from build123d import *
from OCP.BRepFilletAPI import BRepFilletAPI_MakeChamfer

# Parameters (mm, degrees)
SKETCH1_W           = 65
SKETCH1_H           = 64
SKETCH1_W_2         = 44.2
SKETCH1_H_2         = 40
BOSS_EXTRUDE1_DEPTH = 15
SKETCH3_W           = 7
SKETCH3_H           = 11.1
SKETCH4_R           = 9.5
CUT_EXTRUDE2_DEPTH  = 74.986485252
SKETCH5_R           = 4
CUT_EXTRUDE3_DEPTH  = 74.32973476
SKETCH8_R           = 2.15
CUT_EXTRUDE6_DEPTH  = 49.013019068
FILLET1_R           = 20
CHAMFER1_SIZE       = 3
CHAMFER1_SIZE2      = 1.732050808
SKETCH9_W           = 12
SKETCH9_H           = 3


with BuildPart() as part:
    # Sketch1 → Boss-Extrude1 (new body)
    with BuildSketch(Plane(origin=(0, 0, 0), x_dir=(1, 0, 0), z_dir=(0, 1, 0))):
        Rectangle(SKETCH1_W, SKETCH1_H)
        Rectangle(SKETCH1_W_2, SKETCH1_H_2, mode=Mode.SUBTRACT)
    extrude(amount=BOSS_EXTRUDE1_DEPTH)

    # Sketch3 → Cut-Revolve1 (revolve, cut)
    with BuildSketch(Plane(origin=(0, 15, 0), x_dir=(1, 0, 0), z_dir=(0, 1, 0))):
        with Locations((25.6, -5.55)):
            Rectangle(SKETCH3_W, SKETCH3_H)
        with Locations((-25.6, -5.55)):
            Rectangle(SKETCH3_W, SKETCH3_H)
    revolve(axis=Axis((22.1, 15, 0), (1, 0, 0)), mode=Mode.SUBTRACT)

    # Sketch4 → Cut-Extrude2 (cut, through all)
    with BuildSketch(Plane(origin=(32.5, 0, 0), x_dir=(0, 0, -1), z_dir=(1, 0, 0))):
        with Locations((0, 15)):
            Circle(SKETCH4_R)
    extrude(amount=-CUT_EXTRUDE2_DEPTH, mode=Mode.SUBTRACT)

    # Sketch5 → Cut-Extrude3 (cut, through all)
    with BuildSketch(Plane.XY.offset(32)):
        with Locations((0, 15)):
            Circle(SKETCH5_R)
    extrude(amount=-CUT_EXTRUDE3_DEPTH, mode=Mode.SUBTRACT)

    # Sketch8 → Cut-Extrude6 (cut, through all)
    with BuildSketch(Plane(origin=(0, 15, 0), x_dir=(1, 0, 0), z_dir=(0, 1, 0))):
        with Locations((18, 16.5)):
            Circle(SKETCH8_R)
        with Locations((18, -16.5)):
            Circle(SKETCH8_R)
        with Locations((-18, -16.5)):
            Circle(SKETCH8_R)
        with Locations((-18, 16.5)):
            Circle(SKETCH8_R)
        with Locations(Location((9, -27, 0), (0, 0, 270))):
            Circle(SKETCH8_R)
        with Locations(Location((-9, -27, 0), (0, 0, 270))):
            Circle(SKETCH8_R)
        with Locations(Location((-9, 27, 0), (0, 0, 270))):
            Circle(SKETCH8_R)
        with Locations(Location((9, 27, 0), (0, 0, 270))):
            Circle(SKETCH8_R)
    extrude(amount=-CUT_EXTRUDE6_DEPTH, mode=Mode.SUBTRACT)

    # Fillet1
    fillet1_edges = [part.edges().sort_by_distance(p)[0] for p in [
        (-32.5, 7.5, -32),
        (32.5, 7.5, -32),
        (32.5, 7.5, 32),
        (-32.5, 7.5, 32),
    ]]
    fillet(fillet1_edges, radius=FILLET1_R)

    # Chamfer1: one chamfer whose edges measure the first distance from different faces: ONE call of the kernel's chamfer builder (chamfer() names one face for all edges)
    chamfer1_edges_1 = [part.edges().sort_by_distance(p)[0] for p in [
        (22.1, 3.9, 0),
    ]]
    chamfer1_side_1 = [part.faces().sort_by_distance(p)[0] for p in [
        (22.1, 0.427200187, 0),
    ]]
    chamfer1_edges_2 = [part.edges().sort_by_distance(p)[0] for p in [
        (-22.1, 3.9, 0),
    ]]
    chamfer1_side_2 = [part.faces().sort_by_distance(p)[0] for p in [
        (-22.1, 0.427200187, 0),
    ]]
    chamfer1 = BRepFilletAPI_MakeChamfer(part.part.solid().wrapped)
    for e in chamfer1_edges_1:
        chamfer1.Add(CHAMFER1_SIZE, CHAMFER1_SIZE2, e.wrapped, chamfer1_side_1[0].wrapped)  # the first distance lies on this face
    for e in chamfer1_edges_2:
        chamfer1.Add(CHAMFER1_SIZE, CHAMFER1_SIZE2, e.wrapped, chamfer1_side_2[0].wrapped)  # the first distance lies on this face
    add(Compound.cast(chamfer1.Shape()), mode=Mode.REPLACE)

    # Sketch9 → Cut-Revolve2 (revolve, cut)
    with BuildSketch(Plane(origin=(0, 15, 0), x_dir=(1, 0, 0), z_dir=(0, 1, 0))):
        with Locations((-6, -21.5)):
            Rectangle(SKETCH9_W, SKETCH9_H)
        with Locations((-6, 21.5)):
            Rectangle(SKETCH9_W, SKETCH9_H)
    revolve(axis=Axis((0, 15, -29.871415895), (0, 0, 1)), mode=Mode.SUBTRACT)


solid = part.part
Geometry: final body of the model. Coordinates: model frame, mm. A direction names the side the tool comes from. Give positions to 0.01 mm unless a question says otherwise; leave off trailing zeros. Write each loop counter-clockwise with the first axis right and the second up, starting at its lowest first coordinate (ties: lowest second). Pieces come first, ordered by that corner, then holes. Notation, with made-up numbers: M 55,48 L 110,48 A27 ccw 110,79 Z; hole C 11,49 d7. An arc over 180 degrees is marked long. Answer in a Markdown table with one row per item. Add a question column.
(1) Section C-C on x = 9. Return loops of the section in (y, z).
(2) Section A-A on z = 0. Return loops of the section in (x, y), and give its area (3 significant figures).
(3) Section D-D on z = 27. Return loops of the section in (x, y), and give its area (3 significant figures).
(4) First-contact query: pin 1 (5.5 mm diameter, centred on x = 9, z = 27, fed in from +Y); pin 2 (3 mm diameter, centred on x = -16.5, y = 11, fed in from -Z); pin 3 (2 mm diameter, centred on x = -19.5, y = 5.5, fed in from -Z); pin 4 (2 mm diameter, centred on x = -24.5, y = 7, fed in from -Z). Flat tips, straight axial feed; report the tip coordinate or a pass-through.
(5) Reachability of faces 1 (the flat face through (0, 2, -20)), 2 (the flat face through (0, 7, -32)), 3 (the flat face through (29.1, 5, 0)) from +Z, -Z, +X, -X, +Y, -Y: full face, straight path, thin tool, end or side. Return the list, or none.
(6) Section B-B on x = 0. Return loops of the section in (y, z).
(7) Ray query, line 1 (Z direction, x = 1, y = 7.75); line 2 (X direction, y = 7.25, z = 27); line 3 (X direction, y = 8, z = 27.5). Return the intervals inside material, ascending.
(8) Mould query, pull axis Z, two halves, no side actions, for faces 4 (the flat face through (-18, 15, 23)), 5 (the cylindrical face through (26.486, 7.605, 26.297)), 6 (the cylindrical face through (11.13, 7.6, -27.28)). Classes: +Z half, -Z half, draft (parallel to the pull), parting line (faces both ways), or undercut.
Result set:
| question | item | result |
|---|---|---|
| 1 | outline | M 0,-32 L 15,-32 L 15,-29.15 L 0,-29.15 Z; M 0,-24.85 L 15,-24.85 L 15,-23 L 7.06,-23 L 7.06,-20 L 0,-20 Z; M 0,20 L 7.06,20 L 7.06,23 L 15,23 L 15,24.85 L 0,24.85 Z; M 0,29.15 L 15,29.15 L 15,32 L 0,32 Z |
| 2 | outline | M -32.5,0 L -22.1,0 L -22.1,0.9 L -23.83,3.9 L -29.1,3.9 L -29.1,5.5 L -32.5,5.5 Z; M 22.1,0 L 32.5,0 L 32.5,5.5 L 29.1,5.5 L 29.1,3.9 L 23.83,3.9 L 22.1,0.9 Z |
| 2 | area | 86.8 mm^2 |
| 3 | outline | M -25.73,0 L -11.15,0 L -11.15,15 L -25.73,15 Z; M -6.85,0 L 6.85,0 L 6.85,15 L 4,15 A4 cw -4,15 L -6.85,15 Z; M 11.15,0 L 25.73,0 L 25.73,15 L 11.15,15 Z |
| 3 | area | 618 mm^2 |
| 4 | pin 1 | stops at y = 15 |
| 4 | pin 2 | stops at z = -31.84 |
| 4 | pin 3 | stops at z = -31.08 |
| 4 | pin 4 | stops at z = -28.7 |
| 5 | face 1 | +Y, -Y |
| 5 | face 2 | -Z, +X, -X, +Y, -Y |
| 5 | face 3 | +Y |
| 6 | outline | M 0,-32 L 11,-32 L 11,-23 L 3,-23 L 3,-20 L 0,-20 Z; M 0,20 L 3,20 L 3,23 L 11,23 L 11,32 L 0,32 Z |
| 7 | line 1 | z = -32 to -23, 23 to 32 |
| 7 | line 2 | x = -25.73 to -11.15, -6.85 to 6.85, 11.15 to 25.73 |
| 7 | line 3 | x = -25.14 to -11.09, -6.91 to 6.91, 11.09 to 25.14 |
| 8 | face 4 | draft |
| 8 | face 5 | +Z half |
| 8 | face 6 | undercut |
